from build123d import *

# Parameters (mm, degrees)
SKETCH1_W              = 1200
SKETCH1_H              = 2500
BOSS_EXTRUDE1_DEPTH    = 1000
CUT_EXTRUDE1_DEPTH     = 2948.880594597
CUT_EXTRUDE2_START     = -1200
CUT_EXTRUDE2_OUTLINE_R = 250
CUT_EXTRUDE2_DEPTH     = 1200


# Read off the part's stored shape, not the designer's step: Cut-Extrude2
with BuildPart() as part:
    # Sketch1 → Boss-Extrude1 (new body)
    with BuildSketch(Plane(origin=(0, 0, 0), x_dir=(1, 0, 0), z_dir=(0, 1, 0))):
        with Locations((-600, 1250)):
            Rectangle(SKETCH1_W, SKETCH1_H)
    extrude(amount=BOSS_EXTRUDE1_DEPTH)

    # Sketch2 → Cut-Extrude1 (cut, through all)
    with BuildSketch(Plane(origin=(0, 1000, 0), x_dir=(1, 0, 0), z_dir=(0, 1, 0))):
        with BuildLine():
            Line((-900, 1794.983443527), (-900, 2500))
            Line((-900, 2500), (-1200, 2500))
            Line((-1200, 2500), (-1200, 1040))
            ThreePointArc((-1200, 1040), (-1157.592226371, 1261.564683763), (-1036.363636364, 1451.809151015))
            ThreePointArc((-1036.363636364, 1451.809151015), (-935.339811358, 1610.346207058), (-900, 1794.983443527))
        make_face()
        with BuildLine():
            Line((0, 2500), (-300, 2500))
            Line((-300, 2500), (-300, 1794.983443527))
            ThreePointArc((-300, 1794.983443527), (-264.660188642, 1610.346207058), (-163.636363636, 1451.809151015))
            ThreePointArc((-163.636363636, 1451.809151015), (-42.407773629, 1261.564683763), (0, 1040))
            Line((0, 1040), (0, 2500))
        make_face()
        with BuildLine():
            Line((-600, 440), (-600, 1300))
            ThreePointArc((-600, 1300), (-812.132034356, 1212.132034356), (-900, 1000))
            Line((-900, 1000), (-900, 520.384757729))
            ThreePointArc((-900, 520.384757729), (-755.291427062, 460.444504227), (-600, 440))
        make_face()
        with BuildLine():
            ThreePointArc((-300, 1000), (-387.867965644, 1212.132034356), (-600, 1300))
            Line((-600, 1300), (-600, 440))
            ThreePointArc((-600, 440), (-444.708572938, 460.444504227), (-300, 520.384757729))
            Line((-300, 520.384757729), (-300, 1000))
        make_face()
        with BuildLine():
            Line((-600, 0), (-600, 440))
            ThreePointArc((-600, 440), (-755.291427062, 460.444504227), (-900, 520.384757729))
            Line((-900, 520.384757729), (-900, 0))
            Line((-900, 0), (-600, 0))
        make_face()
        with BuildLine():
            ThreePointArc((-300, 520.384757729), (-444.708572938, 460.444504227), (-600, 440))
            Line((-600, 440), (-600, 0))
            Line((-600, 0), (-300, 0))
            Line((-300, 0), (-300, 520.384757729))
        make_face()
    extrude(amount=-CUT_EXTRUDE1_DEPTH, mode=Mode.SUBTRACT)

    # Cut-Extrude2 outline → Cut-Extrude2 (cut)
    with BuildSketch(Plane(origin=(0, 0, 0), x_dir=(0, 0, -1), z_dir=(1, 0, 0)).offset(CUT_EXTRUDE2_START)):
        with BuildLine():
            ThreePointArc((500.000000017, 1000), (682.574185843, 965.474668123), (839.93463424, 866.666666667))
            ThreePointArc((839.93463424, 866.666666667), (918.614858442, 817.262665937), (1009.901951359, 800))
            Line((1009.901951359, 800), (2500, 800))
            Line((2500, 800), (2500, 1000))
            Line((2500, 1000), (500.000000017, 1000))
        make_face()
        with BuildLine():
            ThreePointArc((0, 500), (146.446609413, 853.5533906), (500.000000017, 1000))
            Line((500.000000017, 1000), (0, 1000))
            Line((0, 1000), (0, 500))
        make_face()
        with BuildLine():
            ThreePointArc((499.999999983, 0), (146.446609401, 146.446609412), (0, 500))
            Line((0, 500), (0, 0))
            Line((0, 0), (499.999999983, 0))
        make_face()
        with BuildLine():
            ThreePointArc((839.93463424, 133.333333333), (682.574185828, 34.525331871), (499.999999983, 0))
            Line((499.999999983, 0), (2500, 0))
            Line((2500, 0), (2500, 200))
            Line((2500, 200), (1009.901951359, 200))
            ThreePointArc((1009.901951359, 200), (918.614858442, 182.737334063), (839.93463424, 133.333333333))
        make_face()
        with Locations((500, 500)):
            Circle(CUT_EXTRUDE2_OUTLINE_R)
    extrude(amount=CUT_EXTRUDE2_DEPTH, mode=Mode.SUBTRACT)


solid = part.part
The listing builds one solid part. Answer for the finished solid, in the listing's coordinates (mm). A direction names the side the tool comes from. Round coordinates to 2 decimals unless told otherwise and drop trailing zeros. Loops run counter-clockwise (first coordinate to the right, second up) from the corner with the lowest first, then second, coordinate; pieces in that order, holes last. Notation, with made-up numbers: M 10.5,77.5 L 53.5,77.5 A20 ccw 53.5,114.5 Z; hole C 61.5,86.25 d8. An arc over 180 degrees is marked long. Return JSON: item names as keys, results as strings.
Q1. Find section B-B, the plane z = -472. Determine the outline of the cut face in (x, y).
Results list:
{"outline": "M -1200,0.78 L -900,0.78 L -900,251.57 L -1200,251.57 Z; M -1200,748.43 L -900,748.43 L -900,999.22 L -1200,999.22 Z; M -300,0.78 L 0,0.78 L 0,251.57 L -300,251.57 Z; M -300,748.43 L 0,748.43 L 0,999.22 L -300,999.22 Z"}
Q2. Find section D-D, the plane x = -600. Determine the outline of the cut face in (y, z).
Results list:
{"outline": "M 200,-2500 L 800,-2500 L 800,-1300 L 200,-1300 Z"}
Q3. Find section A-A, the plane y = 598.5. Determine the outline of the cut face in (x, z).
Results list:
{"outline": "M -1200,-1040 A600 ccw -1036.36,-1451.81 A500 cw -900,-1794.98 L -900,-2500 L -300,-2500 L -300,-1794.98 A500 cw -163.64,-1451.81 A600 ccw 0,-1040 L 0,-729.78 L -300,-729.78 L -300,-1000 A300 cw -900,-1000 L -900,-729.78 L -1200,-729.78 Z; M -1200,-270.22 L -900,-270.22 L -900,-9.8 L -1200,-9.8 Z; M -300,-270.22 L 0,-270.22 L 0,-9.8 L -300,-9.8 Z"}
Q4. Each of these flat-tipped pins is pushed along its axis until it touches: pin 1 Ø1 at (x, y) = (-158, 498) entering from -Z; pin 2 Ø5 at (x, z) = (-210, -643) entering from -Y; pin 3 Ø2 at (x, z) = (-407, -1822.5) entering from +Y. Where does it stop, or does it pass through?
Results list:
{"pin 1": "stops at z = -1446.3", "pin 2": "stops at y = 20.15", "pin 3": "stops at y = 800"}
Q5. Find the intervals of material crossed by line 1 along X through (y, z) = (818, -636); line 2 along Y through (x, z) = (-811.5, -2277.5); line 3 along Z through (x, y) = (-1115, 500), in increasing order. Write a range as from..to.
Results list:
{"line 1": "x = -1200..-900, -300..0", "line 2": "y = 200..800", "line 3": "z = -1347.86..-750, -250..0"}
Q6. Which of the six approach directions +Z, -Z, +X, -X, +Y, -Y give full straight-line access (tool end or side, diameter ignored) to faces 1 (the face through (-608, 800, -1745)), 2 (the face through (-900, 504, -2143)), 3 (the face through (-900, 396, -729)), 4 (the face through (-608, 200, -1765))?
Results list:
{"face 1": "-Z, +X, -X, +Y", "face 2": "-Z, -X, +Y, -Y", "face 3": "+Z, +Y, -Y", "face 4": "-Z, +X, -X, -Y"}
Q7. The mould has two halves that part along X. Classify faces 5 (the face through (-300, 396, -271)), 6 (the face through (-593.403, 504.203, -1299.927)), 7 (the face through (-1200, 715, -628)), 8 (the face through (0, 715, -628)): released by +X, released by -X, zero draft, split by the parting line, or undercut.
Results list:
{"face 5": "undercut", "face 6": "undercut", "face 7": "released by -X", "face 8": "released by +X"}
Q8. Find section C-C, the plane y = 391.5. Determine the outline of the cut face in (x, z).
Results list:
{"outline": "M -1200,-1040 A600 ccw -1036.36,-1451.81 A500 cw -900,-1794.98 L -900,-2500 L -300,-2500 L -300,-1794.98 A500 cw -163.64,-1451.81 A600 ccw 0,-1040 L 0,-725.23 L -300,-725.23 L -300,-1000 A300 cw -900,-1000 L -900,-725.23 L -1200,-725.23 Z; M -1200,-274.77 L -900,-274.77 L -900,-11.91 L -1200,-11.91 Z; M -300,-274.77 L 0,-274.77 L 0,-11.91 L -300,-11.91 Z"}
